Autodesk Fusion 360 part; units mm, degrees
sketch "スケッチ1" plane through (0, 0, 0) normal (0, 0, 1) x (1, 0, 0)
  line L0 (0, 0) -> (90, 0)
  line L1 (21.7798, 15.4252) -> (90, 9.4567)
  line L2 (90, 290.5433) -> (21.7798, 284.5748)
  line L3 (0, 300) -> (90, 300)
  line L4 (9, 270.6281) -> (9, 29.3719)
  line L5 (0, 300) -> (0, 0)
  arc A0 (9, 29.3719) -> (21.7798, 15.4252) centre (23, 29.3719) ccw
  arc A1 (21.7798, 284.5748) -> (9, 270.6281) centre (23, 270.6281) ccw
  line L6 (90, 9.4567) -> (90, 0)
  line L7 (90, 300) -> (90, 290.5433)
extrude "押し出し1" add sketch "スケッチ1" along normal blind 100
Here's how the part is built. I have some questions about the finished solid (model axes, mm). A direction names the side the tool comes from. Round coordinates to 2 decimals unless told otherwise and drop trailing zeros. Order: outer loops, then holes, each group sorted by start corner. A loop starts at its lowest first (then second) coordinate and runs counter-clockwise, first axis right, second up. Notation, with made-up numbers: M -27,68.5 L -23,68.5 A16 ccw -23,77.5 Z; hole C -29,-7.5 d11. An arc over 180 degrees is marked long. Return JSON: item names as keys, results as strings. Group by question number.
1. If we mould it in two halves opening along Y, with no side actions, what happens to faces 1 (the face through (44, 0, 49)), 2 (the face through (44, 300, 49)), 3 (the face through (56.37, 287.6, 49.3)), 4 (the face through (90, 295, 49))? For each: pulls with the +Y half, pulls with the -Y half, needs draft (parallel to the pull), parting line crosses it, or undercut.
2. If we section it at B-B on z = 79: List the corners of the cut face in (x, y) for me, then the cut area to 3 significant figures.
3. I'm going to push flat-ended pins straight in: pin 1 Ø6 at (y, z) = (51.5, 32.5) entering from +X; pin 2 Ø3 at (x, y) = (12, 185.5) entering from +Z. Where does each tip first touch, or does it pass through?
4. Please list where these lines run through material, in increasing order: probe 1 along X at (y, z) = (257.5, 9.5); probe 2 along Y at (x, z) = (71.5, 31); probe 3 along Y at (x, z) = (73.5, 77).
5. If we section it at D-D on y = 183: List the corners of the cut face in (x, z) for me, then the cut area to 3 significant figures.
6. On a 3-axis mill with a long thin cutter (end or side, diameter ignored), from which of +Z, -Z, +X, -X, +Y, -Y can I reach the whole of each face in a straight line? I mean faces 5 (the face through (12.6, 280, 49.3)), 6 (the face through (90, 5, 49)). Say none if no direction works.
7. If we section it at C-C on x = 84.5: List the corners of the cut face in (y, z) for me, then the cut area to 3 significant figures.
8. If we section it at A-A on x = 43: List the corners of the cut face in (y, z) for me.
Reply:
{
 "1": {"face 1": "pulls with the -Y half", "face 2": "pulls with the +Y half", "face 3": "undercut", "face 4": "needs draft"},
 "2": {"outline": "M 0,0 L 90,0 L 90,9.46 L 21.78,15.43 A14 cw 9,29.37 L 9,270.63 A14 cw 21.78,284.57 L 90,290.54 L 90,300 L 0,300 Z", "area": "4,870 mm^2"},
 "3": {"pin 1": "x = 9", "pin 2": "through"},
 "4": {"probe 1": "0 to 9", "probe 2": "0 to 11.08, 288.92 to 300", "probe 3": "0 to 10.9, 289.1 to 300"},
 "5": {"outline": "M 0,0 L 9,0 L 9,100 L 0,100 Z", "area": "900 mm^2"},
 "6": {"face 5": "+Z, -Z, +X", "face 6": "+Z, -Z, +X, +Y, -Y"},
 "7": {"outline": "M 0,0 L 9.94,0 L 9.94,100 L 0,100 Z; M 290.06,0 L 300,0 L 300,100 L 290.06,100 Z", "area": "1,990 mm^2"},
 "8": {"outline": "M 0,0 L 13.57,0 L 13.57,100 L 0,100 Z; M 286.43,0 L 300,0 L 300,100 L 286.43,100 Z"}
}
